from build123d import *

# Parameters (mm, degrees)
SKETCH1_W           = 254
SKETCH1_H           = 45.72
BOSS_EXTRUDE1_DEPTH = 5.08
SKETCH2_R           = 17.78
CUT_EXTRUDE2_DEPTH  = 259.131991043
CUT_EXTRUDE3_DEPTH  = 259.131991043
FILLET1_R           = 25.4
SKETCH5_W           = 5.08
SKETCH5_H           = 25.4
BOSS_EXTRUDE2_DEPTH = 5.08
SKETCH7_W           = 5.08
SKETCH7_H           = 19.05
CUT_EXTRUDE4_DEPTH  = 31.75
SKETCH9_W           = 5.08
SKETCH9_H           = 19.05
BOSS_EXTRUDE3_DEPTH = 5.08
SKETCH10_W          = 41.91
SKETCH10_H          = 30.48
CUT_EXTRUDE6_DEPTH  = 260.08


with BuildPart() as part:
    # Sketch1 → Boss-Extrude1 (new body)
    with BuildSketch(Plane(origin=(0, 0, 0), x_dir=(0, 0, -1), z_dir=(1, 0, 0))):
        with Locations((127, 22.86)):
            Rectangle(SKETCH1_W, SKETCH1_H)
    extrude(amount=BOSS_EXTRUDE1_DEPTH)

    # Sketch2 → Cut-Extrude2 (cut, through all)
    with BuildSketch(Plane(origin=(5.08, 0, 0), x_dir=(0, 0, -1), z_dir=(1, 0, 0))):
        with Locations((127, 20.32)):
            Circle(SKETCH2_R)
    extrude(amount=-CUT_EXTRUDE2_DEPTH, mode=Mode.SUBTRACT)

    # Sketch4 → Cut-Extrude3 (cut, through all)
    with BuildSketch(Plane(origin=(5.08, 0, 0), x_dir=(0, 0, -1), z_dir=(1, 0, 0))):
        Polygon((109.22, 20.32), (109.22, 45.72), (127, 45.72), (144.78, 45.72), (144.78, 20.32), align=None)
    extrude(amount=-CUT_EXTRUDE3_DEPTH, mode=Mode.SUBTRACT)

    # Fillet1
    fillet1_edges = [part.edges().sort_by_distance(p)[0] for p in [
        (2.54, 0, -254),
        (2.54, 0, 0),
    ]]
    fillet(fillet1_edges, radius=FILLET1_R)

    # Sketch5 → Boss-Extrude2 (add)
    with BuildSketch(Plane(origin=(0, 45.72, 0), x_dir=(1, 0, 0), z_dir=(0, 1, 0))):
        with Locations((2.54, 54.61)):
            Rectangle(SKETCH5_W, SKETCH5_H)
    extrude(amount=BOSS_EXTRUDE2_DEPTH)

    # Sketch7 → Cut-Extrude4 (cut)
    with BuildSketch(Plane(origin=(5.08, 0, 0), x_dir=(0, 0, -1), z_dir=(1, 0, 0))):
        with Locations((12.7, 36.195)):
            Rectangle(SKETCH7_W, SKETCH7_H)
    cut_extrude4 = extrude(amount=-CUT_EXTRUDE4_DEPTH, mode=Mode.SUBTRACT)

    # Mirror1: Cut-Extrude4 across plane
    add(cut_extrude4.mirror(Plane.XY.offset(-127)), mode=Mode.SUBTRACT)

    # Sketch9 → Boss-Extrude3 (add)
    with BuildSketch(Plane(origin=(0, 45.72, 0), x_dir=(1, 0, 0), z_dir=(0, 1, 0))):
        with Locations((2.54, 229.235)):
            Rectangle(SKETCH9_W, SKETCH9_H)
        with Locations((2.54, 159.385)):
            Rectangle(SKETCH9_W, SKETCH9_H)
    extrude(amount=BOSS_EXTRUDE3_DEPTH)

    # Sketch10 → Cut-Extrude6 (cut, through all)
    with BuildSketch(Plane(origin=(5.08, 0, 0), x_dir=(0, 0, -1), z_dir=(1, 0, 0))):
        with Locations((194.31, 30.48)):
            Rectangle(SKETCH10_W, SKETCH10_H)
    extrude(amount=-CUT_EXTRUDE6_DEPTH, mode=Mode.SUBTRACT)


solid = part.part
Geometry check sheet. Reference: the model listing, model coordinates, mm. A direction names the side the tool comes from. Give positions to 0.01 mm unless a question says otherwise; leave off trailing zeros. Order: outer loops, then holes, each group sorted by start corner. A loop starts at its lowest first (then second) coordinate and runs counter-clockwise, first axis right, second up. Notation, with made-up numbers: M -19,50.25 L 9,50.25 A6 cw 9,59.25 Z; hole C -6.75,-31.75 d5. An arc over 180 degrees is marked long. Use a Markdown table: item, result.
Item 1: Tool access check on faces 4 (the flat face through (3, 36, -10.16)), 5 (the flat face through (3, 45.72, -249)), 6 (the flat face through (3, 50.8, -229)), 7 (the cylindrical face through (2.58, 7.24, -246.36)), 8 (the flat face through (3, 45.72, -28)). Record the directions out of +Z, -Z, +X, -X, +Y, -Y that give a thin tool (end or side, any length) a straight path to the whole face; none if there is none.
Answers follow:
| item | result |
|---|---|
| face 4 | +X, -X, +Y |
| face 5 | -Z, +X, -X, +Y |
| face 6 | +Z, -Z, +X, -X, +Y |
| face 7 | -Z, +X, -X, -Y |
| face 8 | +Z, +X, -X, +Y |
Item 2: Material ranges on line 1 along Z through (x, y) = (3.5, 28) (3 decimals); line 2 along Z through (x, y) = (2.15, 20.5) (3 decimals); line 3 along Z through (x, y) = (1.6, 18) (3 decimals), recorded low to high.
Answers follow:
| item | result |
|---|---|
| line 1 | z = -254 to -243.84, -238.76 to -215.265, -173.355 to -144.78, -109.22 to -15.24, -10.16 to 0 |
| line 2 | z = -253.523 to -215.265, -173.355 to -144.78, -109.22 to -0.477 |
| line 3 | z = -252.898 to -215.265, -173.355 to -144.628, -109.372 to -1.102 |
Item 3: Draft check along Z on faces 1 (the flat face through (3, 36, -15.24)), 2 (the flat face through (5.08, 2, -125)), 3 (the cylindrical face through (2.58, 7.64, -7.24)). Enter one of: +Z half, -Z half, draft (parallel to the pull), parting line (faces both ways), or undercut.
Answers follow:
| item | result |
|---|---|
| face 1 | undercut |
| face 2 | draft |
| face 3 | +Z half |
Item 4: Section check C-C (z = -36). Record the cut outline in (x, y).
Answers follow:
| item | result |
|---|---|
| outline | M 0,0 L 5.08,0 L 5.08,45.72 L 0,45.72 Z |
Item 5: Section check D-D (z = -208.5). Record the cut outline in (x, y), and give its area (3 significant figures).
Answers follow:
| item | result |
|---|---|
| outline | M 0,0 L 5.08,0 L 5.08,15.24 L 0,15.24 Z |
| area | 77.4 mm2 |
Item 6: Depth check by flat-ended pin: P1, Ø1.5, axis at x = 3, y = 48.5, coming from the -Z side; P2, Ø2, axis at x = 2, z = -171, coming from the +Y side; P3, Ø3, axis at x = 1.5, z = -192, coming from the +Y side. Enter the tip coordinate at first touch or a pass-through.
Answers follow:
| item | result |
|---|---|
| P1 | stops at z = -238.76 |
| P2 | stops at y = 45.72 |
| P3 | stops at y = 15.24 |
Item 7: Section check A-A (y = 43.5). Record the cut outline in (x, z) (3 decimals), and give its area (3 significant figures).
Answers follow:
| item | result |
|---|---|
| outline | M 0,-254 L 5.08,-254 L 5.08,-243.84 L 0,-243.84 Z; M 0,-238.76 L 5.08,-238.76 L 5.08,-215.265 L 0,-215.265 Z; M 0,-173.355 L 5.08,-173.355 L 5.08,-144.78 L 0,-144.78 Z; M 0,-109.22 L 5.08,-109.22 L 5.08,-15.24 L 0,-15.24 Z; M 0,-10.16 L 5.08,-10.16 L 5.08,0 L 0,0 Z |
| area | 845 mm2 |
